```python
from build123d import *

# Parameters (mm, degrees)
F0_W     = 130
F0_H     = 250
F0_R     = 14
F1_DEPTH = 10
F5_DEPTH = 130


with BuildPart() as f1:
    # F0 (on Front) → F1 (new body, symmetric)
    with BuildSketch(Plane.XZ):
        Rectangle(F0_W, F0_H)
        with Locations((0, 75)):
            Circle(F0_R, mode=Mode.SUBTRACT)
    extrude(amount=F1_DEPTH, both=True)

    # F4 (on face) → F5 (join)
    with BuildSketch(Plane.YZ.offset(65)):
        Polygon((-10, 125), (10, 125), (10, 130), align=None)
    extrude(amount=-F5_DEPTH)


solid = f1.part
```
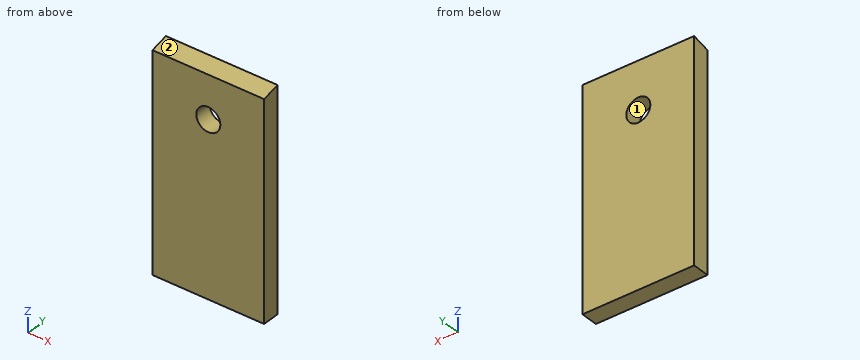
Source: CAD feature listing. Evaluate the final solid. Frame: model axes, mm. Face numbers are marked on the shaded views. Round coordinates to 2 decimals unless told otherwise and drop trailing zeros. Write each loop counter-clockwise with the first axis right and the second up, starting at its lowest first coordinate (ties: lowest second). Pieces come first, ordered by that corner, then holes. Notation, with made-up numbers: M 44.25,39.25 L 98.25,39.25 A21 cw 98.25,43.25 Z; hole C 39.25,-9.5 d9. An arc over 180 degrees is marked long. Answer as a JSON object with one key per item and string values. Group by question number.
(1) Ray query, line 1 (X direction, y = -4.5, z = 74); line 2 (Z direction, x = 0, y = -3.5) (3 decimals); line 3 (Z direction, x = 0, y = 4.25). Return the intervals inside material, ascending. Write a range as [from, to].
(2) Section query C-C on y = -3.25. Output: boundary loops of the cut face in (x, z).
(3) Section query A-A on z = 75. Output: boundary loops of the cut face in (x, y), then the cut area to 3 significant figures.
(4) Mould query, pull axis X, two halves, no side actions, for the marked faces 1 and 2. Classes: +X half, -X half, draft (parallel to the pull), parting line (faces both ways), or undercut.
(5) First-contact query: pin 1 (6 mm diameter, centred on x = 24, y = 3.5, fed in from +Z) (3 decimals); pin 2 (1 mm diameter, centred on x = -32, y = 1.5, fed in from +Z); pin 3 (1 mm diameter, centred on x = 38, y = 2, fed in from +Z) (3 decimals). Flat tips, straight axial feed; report the tip coordinate or a pass-through.
(6) Section query B-B on x = 0. Output: boundary loops of the cut face in (y, z).
Computed values:
{
 "1": {"line 1": "[-65, -13.96], [13.96, 65]", "line 2": "[-125, 61], [89, 126.625]", "line 3": "[-125, 61], [89, 128.56]"},
 "2": {"outline": "M -65,-125 L 65,-125 L 65,126.69 L -65,126.69 Z; hole C 0,75 d28"},
 "3": {"outline": "M -65,-10 L -14,-10 L -14,10 L -65,10 Z; M 14,-10 L 65,-10 L 65,10 L 14,10 Z", "area": "2,040 mm^2"},
 "4": {"face 1": "undercut", "face 2": "draft"},
 "5": {"pin 1": "z = 129.125", "pin 2": "z = 128", "pin 3": "z = 128.125"},
 "6": {"outline": "M -10,-125 L 10,-125 L 10,61 L -10,61 Z; M -10,89 L 10,89 L 10,130 L -10,125 Z"}
}
